Drawing for the job (mm, zero at the part's lowest x, y, z). Coordinates: 2 decimals unless noted, no trailing zeros. Order: outer loops, then holes, each group sorted by start corner. A loop starts at its lowest first (then second) coordinate and runs counter-clockwise, first axis right, second up. Notation, with made-up numbers: (-37.75, 56) - (7.25, 56) arc R36 cw to (7.25, 91) - close; hole circle Ø4 at (22, -4). An arc over 180 degrees is marked (long way). Answer as CSV lines item,"result". Start each with the question number.
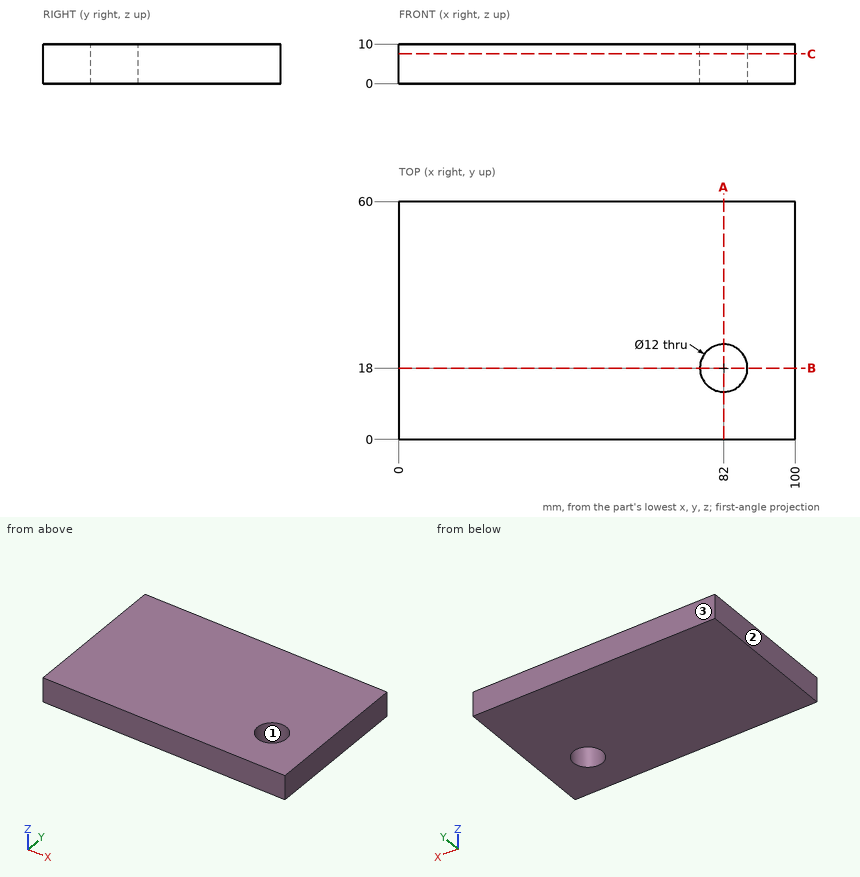
(1) Band-saw the part on B-B on y = 18. List the corners of the cut face in (x, z), plus the area to 3 significant figures.
(2) Drop a flat-ended pin along its axis: pin 1 Ø9.5 at (x, y) = (82, 18) entering from +Z. Give the stop position or say it passes through.
(3) Band-saw the part on C-C on z = 7.5. List the corners of the cut face in (x, y).
(4) Probe L1, parallel to Y at x = 81.5, z = 5; L2, parallel to Y at x = 83, z = 7.75; L3, parallel to X at y = 16, z = 6.75. List the from-to ranges inside material, lowest first. Write a range as [from, to].
(5) Band-saw the part on A-A on x = 82. List the corners of the cut face in (y, z).
(6) Pull direction Y, two halves, no side cores. Call the marked faces 1, 2 and 3: +Y half, -Y half, draft (parallel to the pull), parting line (faces both ways), or undercut.
Filled in:
1,outline,"(0, 0) - (76, 0) - (76, 10) - (0, 10) - close; (88, 0) - (100, 0) - (100, 10) - (88, 10) - close"
1,area,"880 mm^2"
2,pin 1,"passes through"
3,outline,"(0, 0) - (100, 0) - (100, 60) - (0, 60) - close; hole circle Ø12 at (82, 18)"
4,L1,"y = [0, 12.02], [23.98, 60]"
4,L2,"y = [0, 12.08], [23.92, 60]"
4,L3,"x = [0, 76.34], [87.66, 100]"
5,outline,"(0, 0) - (12, 0) - (12, 10) - (0, 10) - close; (24, 0) - (60, 0) - (60, 10) - (24, 10) - close"
6,face 1,"undercut"
6,face 2,"draft"
6,face 3,"+Y half"
